Input: part model. Units: mm. Frame: model coordinates. A direction names the side the tool comes from. Give positions to 0.01 mm unless a question says otherwise; leave off trailing zeros. Loops run counter-clockwise (first coordinate to the right, second up) from the corner with the lowest first, then second, coordinate; pieces in that order, holes last. Notation, with made-up numbers: (-6, 0.25) - (46, 0.25) arc R20 cw to (46, 7.25) - close; hole circle Ø1 at (21.5, -6.75). An arc over 180 degrees is marked (long way). One line per item, written item: value.
from build123d import *

# Parameters (mm, degrees)
SKETCH1_W           = 10
SKETCH1_H           = 30
BOSS_EXTRUDE1_DEPTH = 10
FILLET2_R           = 1
SKETCH2_W           = 8
SKETCH2_H           = 8
CUT_EXTRUDE1_DEPTH  = 28
SKETCH4_R           = 1.5
CUT_EXTRUDE2_DEPTH  = 8
CUT_EXTRUDE3_DEPTH  = 19.708286934
LPATTERN1_COUNT     = 4
LPATTERN1_PITCH     = 7
CUT_EXTRUDE4_DEPTH  = 19.708286934
LPATTERN2_COUNT     = 3
LPATTERN2_PITCH     = 7
SKETCH7_W           = 8
SKETCH7_H           = 1
BOSS_EXTRUDE2_DEPTH = 3
FILLET4_R           = 3
LPATTERN3_COUNT     = 2
LPATTERN3_PITCH     = 7
FILLET5_R           = 3
SKETCH8_R           = 1
CUT_EXTRUDE5_DEPTH  = 21.736441353


with BuildPart() as part:
    # Sketch1 → Boss-Extrude1 (new body)
    with BuildSketch(Plane.XY):
        Rectangle(SKETCH1_W, SKETCH1_H)
    extrude(amount=BOSS_EXTRUDE1_DEPTH)

    # Fillet2
    fillet2_edges = [part.edges().sort_by_distance(p)[0] for p in [
        (5, 0, 10),
        (0, 15, 10),
        (-5, 0, 10),
        (0, 15, 0),
        (5, 0, 0),
        (0, -15, 0),
        (-5, 0, 0),
        (-5, 15, 5),
        (5, 15, 5),
        (5, -15, 5),
        (-5, -15, 5),
        (0, -15, 10),
    ]]
    fillet(fillet2_edges, radius=FILLET2_R)

    # Sketch2 → Cut-Extrude1 (cut)
    with BuildSketch(Plane(origin=(0, 14, 0), x_dir=(1, 0, 0), z_dir=(0, 1, 0))):
        with Locations((0, -5)):
            Rectangle(SKETCH2_W, SKETCH2_H)
    extrude(amount=-CUT_EXTRUDE1_DEPTH, mode=Mode.SUBTRACT)

    # Sketch4 → Cut-Extrude2 (cut)
    with BuildSketch(Plane(origin=(0, 15, 0), x_dir=(1, 0, 0), z_dir=(0, 1, 0))):
        with Locations(Location((0, -5, 0), (0, 0, 270))):
            Circle(SKETCH4_R)
    extrude(amount=-CUT_EXTRUDE2_DEPTH, mode=Mode.SUBTRACT)

    # Sketch5 → Cut-Extrude3 (cut, through all)
    with BuildSketch(Plane.XY.offset(10)):
        with BuildLine():
            Line((-2.263626959, 12.736789234), (1.510119058, 10.712247379))
            ThreePointArc((1.510119058, 10.712247379), (1.773609184, 10.283344823), (1.530469097, 9.842587126))
            Line((1.530469097, 9.842587126), (-2.24327692, 7.584614681))
            ThreePointArc((-2.24327692, 7.584614681), (-2.746615551, 7.578726428), (-3, 8.013675586))
            Line((-3, 8.013675586), (-3, 12.296189886))
            ThreePointArc((-3, 12.296189886), (-2.75672308, 12.725250791), (-2.263626959, 12.736789234))
        make_face()
    cut_extrude3 = extrude(amount=-CUT_EXTRUDE3_DEPTH, mode=Mode.SUBTRACT)

    # LPattern1: Cut-Extrude3 ×4
    with Locations(*[(0, -i * LPATTERN1_PITCH, 0) for i in range(1, LPATTERN1_COUNT)]):
        add(cut_extrude3, mode=Mode.SUBTRACT)

    # Sketch6 → Cut-Extrude4 (cut, through all)
    with BuildSketch(Plane(origin=(0, 0, 0), x_dir=(-1, 0, 0), z_dir=(0, 0, -1))):
        with BuildLine():
            Line((-1.773746018, 8.053772264), (-1.773746018, 5.671291651))
            ThreePointArc((-1.773746018, 5.671291651), (-1.5114064, 5.231385363), (-0.999675848, 5.253098463))
            Line((-0.999675848, 5.253098463), (0.817992167, 6.44433877))
            ThreePointArc((0.817992167, 6.44433877), (1.043921997, 6.862531957), (0.817992167, 7.280725145))
            Line((0.817992167, 7.280725145), (-0.999675848, 8.471965452))
            ThreePointArc((-0.999675848, 8.471965452), (-1.5114064, 8.493678552), (-1.773746018, 8.053772264))
        make_face()
    cut_extrude4 = extrude(amount=-CUT_EXTRUDE4_DEPTH, mode=Mode.SUBTRACT)

    # LPattern2: Cut-Extrude4 ×3
    with Locations(*[(0, -i * LPATTERN2_PITCH, 0) for i in range(1, LPATTERN2_COUNT)]):
        add(cut_extrude4, mode=Mode.SUBTRACT)

    # Sketch7 → Boss-Extrude2 (add)
    with BuildSketch(Plane.XZ.offset(15)):
        with Locations((0, 8.5)):
            Rectangle(SKETCH7_W, SKETCH7_H)
    boss_extrude2 = extrude(amount=BOSS_EXTRUDE2_DEPTH)

    # Fillet4
    fillet4_edges = [part.edges().sort_by_distance(p)[0] for p in [
        (4, -18, 8.5),
        (-4, -18, 8.5),
    ]]
    fillet(fillet4_edges, radius=FILLET4_R - 0.0001)  # a hair under: the kernel refuses the full size

    # LPattern3: Boss-Extrude2 ×2
    with Locations(*[(0, 0, -i * LPATTERN3_PITCH) for i in range(1, LPATTERN3_COUNT)]):
        add(boss_extrude2)

    # Fillet5
    fillet5_edges = [part.edges().sort_by_distance(p)[0] for p in [
        (4, -18, 1.5),
        (-4, -18, 1.5),
    ]]
    fillet(fillet5_edges, radius=FILLET5_R - 0.0001)  # a hair under: the kernel refuses the full size

    # Sketch8 → Cut-Extrude5 (cut, through all)
    with BuildSketch(Plane.XY.offset(9)):
        with Locations((0, -16.338268511)):
            Circle(SKETCH8_R)
    extrude(amount=-CUT_EXTRUDE5_DEPTH, mode=Mode.SUBTRACT)


solid = part.part
Item 1: Section C-C, the plane x = 3. Output: boundary loops of the cut face in (y, z), and give its area (3 significant figures).
Verdict:
outline: (-17.24, 1) - (-15, 1) arc R1 ccw to (-14, 0) - (14, 0) arc R1 ccw to (15, 1) - (15, 9) arc R1 ccw to (14, 10) - (-14, 10) arc R1 ccw to (-15, 9) - (-17.24, 9) - (-17.24, 8) - (-15, 8) - (-15, 2) - (-17.24, 2) - close; hole (-14, 1) - (14, 1) - (14, 9) - (-14, 9) - close
area: 79.6 mm^2
Item 2: Section A-A, the plane z = 5. Output: boundary loops of the cut face in (x, y), and give its area (3 significant figures).
Verdict:
outline: (-5, -14) arc R1 ccw to (-4, -15) - (4, -15) arc R1 ccw to (5, -14) - (5, 14) arc R1 ccw to (4, 15) - (1.5, 15) - (1.5, 14) - (4, 14) - (4, -14) - (-4, -14) - (-4, 14) - (-1.5, 14) - (-1.5, 15) - (-4, 15) arc R1 ccw to (-5, 14) - close
area: 72.1 mm^2
Item 3: Section B-B, the plane y = -3. Output: boundary loops of the cut face in (x, z), and give its area (3 significant figures).
Verdict:
outline: (-5, 1) arc R1 ccw to (-4, 0) - (-3, 0) - (-3, 1) - (-4, 1) - (-4, 9) - (-3, 9) - (-3, 10) - (-4, 10) arc R1 ccw to (-5, 9) - close; (0.97, 0) - (4, 0) arc R1 ccw to (5, 1) - (5, 9) arc R1 ccw to (4, 10) - (0.97, 10) - (0.97, 9) - (4, 9) - (4, 1) - (0.97, 1) - close
area: 27.2 mm^2
Item 4: Draft query along X for faces 1 (the face through (-0.403, 11.739, 9.507)), 2 (the face through (-1, -17, 8)), 3 (the face through (3.1, -17.14, 8.51)). Return one class per face: pulls with the +X half, pulls with the -X half, needs draft (parallel to the pull), parting line crosses it, or undercut.
Verdict:
face 1: undercut
face 2: needs draft
face 3: pulls with the +X half
Item 5: Pin query (flat end, axial travel): P1, Ø0.8, axis at y = -7, z = 0.5, coming from the -X side (3 decimals); P2, Ø2.5, axis at x = 0, y = -16.34, coming from the -Z side; P3, Ø0.9, axis at x = -1.5, y = -16, coming from the +Z side. Return the tip coordinate at first contact, or that it passes through.
Verdict:
P1: stops at x = -4.995
P2: stops at z = 1
P3: stops at z = 9
Item 6: Material intervals for L1, parallel to Y at x = 0, z = 1.7; L2, parallel to X at y = -9.5, z = 2.5; L3, parallel to Y at x = 2.5, z = 3.75, sorted ascending.
Verdict:
L1: y = -18 to -17.34, -15.34 to -14, 14 to 15
L2: x = -5 to -4, 4 to 5
L3: y = -15 to -14, 14 to 15
Item 7: Section D-D, the plane z = 1.5. Count the separate pieces of the cut face and the enclosed holes in it, and give its area (3 significant figures).
Verdict:
separate pieces: 1
enclosed holes: 2
area: 92.1 mm^2
Item 8: Access query for faces 4 (the face through (0, -15, 5)), 5 (the face through (-2, 14, 5)), 6 (the face through (0.08, 7.87, 9.49)). Directions: +Z, -Z, +X, -X, +Y, -Y. A direction counts if a zero-diameter tool reaches every point of the face in a straight line with its end or side. Return the directions, or none.
Verdict:
face 4: +X, -X, -Y
face 5: none
face 6: +Z, -Z
